The listing builds one solid part. Answer for the finished solid, in the listing's coordinates (mm). A direction names the side the tool comes from. Round coordinates to 2 decimals unless told otherwise and drop trailing zeros. Order: outer loops, then holes, each group sorted by start corner. A loop starts at its lowest first (then second) coordinate and runs counter-clockwise, first axis right, second up. Notation, with made-up numbers: M 35.25,29 L 84.25,29 A15 ccw 84.25,39 Z; hole C 5,61.5 d7. An arc over 180 degrees is marked long. Put each result on its own line as item: value. Start each with the question number.
1. Consider line 1 (Z direction, x = 0, y = 14.5); line 2 (Z direction, x = -5, y = 0); line 3 (Y direction, x = -2.75, z = 0). Determine where each line is inside the solid, lowest interval first.
2. The mould has two halves that part along X. Classify faces 4 (the face through (-3.1, 11.43, -3.1)), 5 (the face through (11.546, 15.195, 0.508)), 6 (the face through (-5.635, -3.997, 1.259)): +X half, -X half, draft (parallel to the pull), parting line (faces both ways), or undercut.
3. Which of the six approach directions +Z, -Z, +X, -X, +Y, -Y give full straight-line access (tool end or side, diameter ignored) to faces 1 (the face through (7.21, 2.83, 0.25)), 2 (the face through (1.542, 16.188, -6.943)), 3 (the face through (-11.43, -3.1, -3.1))?
4. Each of these flat-tipped pins is pushed along its axis until it touches: pin 1 Ø12 at (y, z) = (17, -0.5) entering from -X; pin 2 Ø13 at (y, z) = (0, 0) entering from +X; pin 3 Ø8.5 at (x, z) = (0, 0) entering from +Y. Where does it stop, or does it pass through?
5. The part is cut by section B-B (x = -12). Give the vertices of the cut face in (y, z), then the cut area to 3 significant figures.
from build123d import *

# Parameters (mm, degrees)
CIRPATTERN2_COUNT  = 2
CIRPATTERN2_ANGLE  = 90
SKETCH4_R          = 4.191
CUT_EXTRUDE1_DEPTH = 22.082
SKETCH5_R          = 4.191
CUT_EXTRUDE2_DEPTH = 22.082
REVOLVE2_ANGLE     = 90


with BuildPart() as part:
    # Sketch2 → Revolve1 (revolve)
    with BuildSketch(Plane.XY):
        with BuildLine():
            Line((-21.082, -7.112), (-11.43, -7.112))
            Line((-11.43, -7.112), (-11.43, -4.191))
            Line((-11.43, -4.191), (0, -4.191))
            Line((0, -4.191), (0, -7.2136))
            Line((0, -7.2136), (-5.5753, -7.2136))
            Line((-5.5753, -7.2136), (-9.9187, -11.557))
            Line((-9.9187, -11.557), (-20.32635, -11.557))
            ThreePointArc((-20.32635, -11.557), (-20.860675239, -11.335675239), (-21.082, -10.80135))
            Line((-21.082, -10.80135), (-21.082, -7.112))
        make_face()
    revolve(axis=Axis((0, 0, 0), (-1, 0, 0)))


with BuildPart() as cirpattern2_1:
    # CirPattern2: pattern copy
    add(part.part.rotate(Axis((0, 0, -11.557), (0, 0, -1)), 1 * CIRPATTERN2_ANGLE / (CIRPATTERN2_COUNT - 1)))

    # Sketch4 → Cut-Extrude1 (cut, through all)
    with BuildSketch(Plane(origin=(0, 0, 0), x_dir=(0, 0, -1), z_dir=(1, 0, 0))):
        Circle(SKETCH4_R)
    extrude(amount=-CUT_EXTRUDE1_DEPTH, mode=Mode.SUBTRACT)


with BuildPart() as part_1:
    add(part.part)

    # Sketch5 → Cut-Extrude2 (cut, through all)
    with BuildSketch(Plane.XZ):
        Circle(SKETCH5_R)
    extrude(amount=-CUT_EXTRUDE2_DEPTH, mode=Mode.SUBTRACT)

    # Combine1: union CirPattern2_1
    add(cirpattern2_1.part)

    # Sketch6 → Revolve2 (revolve)
    with BuildSketch(Plane(origin=(0, 0, 0), x_dir=(0, 0, -1), z_dir=(1, 0, 0))):
        with BuildLine():
            Line((-7.2136, 0), (-4.191, 0))
            ThreePointArc((-4.191, 0), (0, -4.191), (4.191, 0))
            Line((4.191, 0), (7.2136, 0))
            ThreePointArc((7.2136, 0), (0, -7.2136), (-7.2136, 0))
        make_face()
    revolve(axis=Axis((0, 0, 4.191), (0, 0, 1)), revolution_arc=REVOLVE2_ANGLE)


solid = part_1.part
Resolved:
1. line 1: -11.56 to -7.11, 7.11 to 11.56
1. line 2: -7.21 to -4.19, 4.19 to 7.21
1. line 3: -7.21 to -4.19
2. face 4: undercut
2. face 5: parting line
2. face 6: draft
3. face 1: none
3. face 2: +Y
3. face 3: -X
4. pin 1: x = -21.05
4. pin 2: x = 8.14
4. pin 3: y = 11.43
5. outline: C 0,0 d23.11; hole C 0,0 d14.22
5. area: 261 mm2
